Input: part model. Units: mm. Frame: model coordinates. A direction names the side the tool comes from. Coordinates: 2 decimals unless noted, no trailing zeros. Order: outer loops, then holes, each group sorted by start corner. A loop starts at its lowest first (then second) coordinate and runs counter-clockwise, first axis right, second up. Notation, with made-up numbers: (20, -1.75) -> (26, -1.75) arc R10 cw to (26, 11.25) -> close; hole circle Ø10 at (9.5, 51). An arc over 180 degrees is marked (long way). One line per item, written item: value. Start each with the question number.
from build123d import *

# Parameters (mm, degrees)
F0_W     = 48
F0_H     = 15
F0_R     = 1
F1_DEPTH = 25
F2_R     = 5
F3_W     = 15
F3_H     = 25
F4_DEPTH = 5


with BuildPart() as f1:
    # F0 (on Front) → F1 (new body)
    with BuildSketch(Plane.XZ):
        with Locations((24, -7.5)):
            Rectangle(F0_W, F0_H)
        with Locations((5, -10)):
            Circle(F0_R, mode=Mode.SUBTRACT)
        with Locations((43, -10)):
            Circle(F0_R, mode=Mode.SUBTRACT)
    extrude(amount=F1_DEPTH)

    # F2
    f2_edges = [f1.edges().sort_by_distance(p)[0] for p in [
        (0, -12.5, -15),
        (48, -12.5, -15),
    ]]
    fillet(f2_edges, radius=F2_R)

    # F3 (on face) → F4 (cut)
    with BuildSketch(Plane.XY):
        with Locations((17.5, -12.5)):
            Rectangle(F3_W, F3_H)
    extrude(amount=-F4_DEPTH, mode=Mode.SUBTRACT)


solid = f1.part
1) Access query for faces 1 (the flat face through (17, -12, -5)), 2 (the flat face through (36, -12, 0)). Directions: +Z, -Z, +X, -X, +Y, -Y. A direction counts if a zero-diameter tool reaches every point of the face in a straight line with its end or side. Return the directions, or none.
2) Section query C-C, the plane x = 13.5. Return the cut outline in (y, z), plus the area to 3 significant figures.
3) Ray query, line 1 along Z through (x, y) = (43, -4.25); line 2 along X through (y, z) = (-13.25, -1); line 3 along X through (y, z) = (-23, -9.75). Return the intervals inside material, ascending. Write a range as from..to.
4) Section query D-D, the plane x = 45.5. Return the cut outline in (y, z).
5) Section query B-B, the plane y = -18.75. Return the cut outline in (x, z).
6) Mould query, pull axis X, two halves, no side actions, for faces 3 (the flat face through (25, -13, -2)), 4 (the flat face through (24, -25, -7)), 5 (the flat face through (48, -12, -5)). Classes: +X half, -X half, draft (parallel to the pull), parting line (faces both ways), or undercut.
7) Pin query (flat end, axial travel): pin 1 Ø2 at (y, z) = (-22, -13) entering from +X; pin 2 Ø7.5 at (x, y) = (15, -11.5) entering from +Z. Return the tip coordinate at first contact, or that it passes through.
8) Section query A-A, the plane z = -0.75. Return the cut outline in (x, y).
Entries:
1. face 1: +Z, +Y, -Y
1. face 2: +Z, +X, -X, +Y, -Y
2. outline: (-25, -15) -> (0, -15) -> (0, -5) -> (-25, -5) -> close
2. area: 250 mm2
3. line 1: z = -15..-11, -9..0
3. line 2: x = 0..10, 25..48
3. line 3: x = 0..4.03, 5.97..42.03, 43.97..48
4. outline: (-25, -14.33) -> (0, -14.33) -> (0, 0) -> (-25, 0) -> close
5. outline: (0, -10) arc R5 ccw to (5, -15) -> (43, -15) arc R5 ccw to (48, -10) -> (48, 0) -> (25, 0) -> (25, -5) -> (10, -5) -> (10, 0) -> (0, 0) -> close; hole circle Ø2 at (5, -10); hole circle Ø2 at (43, -10)
6. face 3: undercut
6. face 4: draft
6. face 5: +X half
7. pin 1: stops at x = 47.58
7. pin 2: stops at z = -5
8. outline: (0, -25) -> (10, -25) -> (10, 0) -> (0, 0) -> close; (25, -25) -> (48, -25) -> (48, 0) -> (25, 0) -> close
